Autodesk Inventor part; units mm, degrees
ref_plane "YZ Plane" through (0, 0, 0) normal (1, 0, 0) x (0, 1, 0)
ref_plane "XZ Plane" through (0, 0, 0) normal (0, 1, 0) x (-1, 0, 0)
ref_plane "XY Plane" through (0, 0, 0) normal (0, 0, 1) x (1, 0, 0)
sketch "Skizze1" plane through (0, 0, 0) normal (0, 0, 1) x (1, 0, 0)
  circle A0 centre (0, 0) radius 19.5
  circle A1 centre (0, 0) radius 21
  dimension "d0" = 39
  dimension "d1" = 42
extrude "Extrusion1" add sketch "Skizze1" along normal blind 8 draft -2
sketch "Skizze2" plane through (0, 0, 0) normal (0, 0, -1) x (-1, 0, 0)
  circle A0 centre (0, 0) radius 19.6
  circle A1 centre (0, 0) radius 21
  circle A2 centre (0, 0) radius 18
  dimension "d4" = 36
extrude "Extrusion2" add sketch "Skizze2" along normal blind 1 contours A0 | A1
properties part number "00_Berrybase_CCTVLens_adapterring_50mm_to_100mm"
Input: part model. Units: mm. Frame: model coordinates. A direction names the side the tool comes from. Round coordinates to 2 decimals unless told otherwise and drop trailing zeros. Order: outer loops, then holes, each group sorted by start corner. A loop starts at its lowest first (then second) coordinate and runs counter-clockwise, first axis right, second up. Notation, with made-up numbers: (74, -10.5) - (95, -10.5) arc R26 ccw to (95, 6.5) - close; hole circle Ø9 at (-17.5, 1.25). An arc over 180 degrees is marked (long way). Answer in a Markdown table with one row per item.
Item 1: Section query C-C (z = 5). Return the cut outline in (x, y).
Model answer:
| item | result |
|---|---|
| outline | circle Ø41.65 at (0, 0); hole circle Ø39.35 at (0, 0) |
Item 2: Reachability of faces 1 (the flat face through (11, -17, 8)), 2 (the flat face through (-5.69, -17.24, 0)) from +Z, -Z, +X, -X, +Y, -Y: full face, straight path, thin tool, end or side. Return the list, or none.
Model answer:
| item | result |
|---|---|
| face 1 | +Z, +X, -X, +Y, -Y |
| face 2 | +Z |
Item 3: Line query: line 1 (Y direction, x = 0, z = -0.6); line 2 (Y direction, x = -17.5, z = 4.5); line 3 (X direction, y = -6.5, z = 4.5). Output: solid intervals per line, ascending.
Model answer:
| item | result |
|---|---|
| line 1 | y = -21 to -18, 18 to 21 |
| line 2 | y = -11.32 to -8.95, 8.95 to 11.32 |
| line 3 | x = -19.8 to -18.55, 18.55 to 19.8 |
Item 4: Pin query (flat end, axial travel): pin 1 (19.5 mm diameter, centred on x = 2.5, y = -4, fed in from +Z); pin 2 (1 mm diameter, centred on x = -8, y = -16, fed in from -Z); pin 3 (2 mm diameter, centred on y = 13, z = 5, fed in from -X); pin 4 (2 mm diameter, centred on y = 1, z = 3, fed in from +X). Return the tip coordinate at first contact, or that it passes through.
Model answer:
| item | result |
|---|---|
| pin 1 | passes through |
| pin 2 | stops at z = -1 |
| pin 3 | stops at x = -17.02 |
| pin 4 | stops at x = 20.92 |
Item 5: Section query A-A (y = 0). Return the cut outline in (x, z), then the cut area to 3 significant figures.
Model answer:
| item | result |
|---|---|
| outline | (-21, -1) - (-18, -1) - (-18, 0) - (-19.5, 0) - (-19.78, 8) - (-20.72, 8) - (-21, 0) - close; (18, -1) - (21, -1) - (21, 0) - (20.72, 8) - (19.78, 8) - (19.5, 0) - (18, 0) - close |
| area | 25.5 mm² |
